Read the model definition and answer for the solid it produces. Units are mm, in the model's axes. A direction names the side the tool comes from. Round coordinates to 2 decimals unless told otherwise and drop trailing zeros. Loops run counter-clockwise (first coordinate to the right, second up) from the corner with the lowest first, then second, coordinate; pieces in that order, holes last. Notation, with made-up numbers: M 13.5,-17.5 L 31.5,-17.5 A18 cw 31.5,-7.5 Z; hole C 72,84 d8. An arc over 180 degrees is marked long. Answer as CSV lines item,"result".
```python
from build123d import *

# Parameters (mm, degrees)
SKETCH_1_R      = 8
EXTRUDE_1_DEPTH = 24
SKETCH_2_R      = 22
SKETCH_2_R_2    = 8
EXTRUDE_2_DEPTH = 18


with BuildPart() as part:
    # 草图1 → 凸台-拉伸1 (new body)
    with BuildSketch(Plane.XY):
        Circle(SKETCH_1_R)
        with BuildLine():
            Line((4.520101179, 2.361924075), (-4.833937562, 1.62574526))
            ThreePointArc((-4.833937562, 1.62574526), (0.400141388, -5.084278402), (4.520101179, 2.361924075))
        make_face(mode=Mode.SUBTRACT)
    extrude(amount=EXTRUDE_1_DEPTH)

    # 草图2 → 凸台-拉伸2 (add)
    with BuildSketch(Plane.XY):
        Circle(SKETCH_2_R)
        Circle(SKETCH_2_R_2, mode=Mode.SUBTRACT)
    extrude(amount=EXTRUDE_2_DEPTH)


solid = part.part
```
1) Find section C-C, the plane z = 5. Give the vertices of the cut face in (x, y).
Evaluation:
outline,"C 0,0 d44; hole M -4.83,1.63 A5.1 ccw long 4.52,2.36 Z"
2) Find section A-A, the plane y = 0. Give the vertices of the cut face in (x, z).
Evaluation:
outline,"M -22,0 L -5.1,0 L -5.1,24 L -8,24 L -8,18 L -22,18 Z; M 5.1,0 L 22,0 L 22,18 L 8,18 L 8,24 L 5.1,24 Z"
3) Find section D-D, the plane x = -6. Give the vertices of the cut face in (y, z), then the cut area to 3 significant figures.
Evaluation:
outline,"M -21.17,0 L 21.17,0 L 21.17,18 L 5.29,18 L 5.29,24 L -5.29,24 L -5.29,18 L -21.17,18 Z"
area,"825 mm^2"
4) Each of these flat-tipped pins is pushed along its axis until it touches: P1, Ø1, axis at y = 6, z = 17, coming from the +X side; P2, Ø1.5, axis at x = -10.5, z = 7, coming from the +Y side; P3, Ø5, axis at x = 15, y = 17, coming from the +Z side. Where does it stop, or does it pass through?
Evaluation:
P1,"stops at x = 21.3"
P2,"stops at y = 19.72"
P3,"stops at z = 18"
5) Straight lines are drawn through the part: line 1 (Z direction, x = -9.5, y = -4); line 2 (Y direction, x = 0, z = 5.5); line 3 (Y direction, x = -3, z = 20). For each, find the intervals that lie inside material, in ascending order.
Evaluation:
line 1,"z = 0 to 18"
line 2,"y = -22 to -5.1, 2.01 to 22"
line 3,"y = -7.42 to -4.12, 1.77 to 7.42"
6) Find section B-B, the plane x = 0. Give the vertices of the cut face in (y, z).
Evaluation:
outline,"M -22,0 L -5.1,0 L -5.1,24 L -8,24 L -8,18 L -22,18 Z; M 2.01,0 L 22,0 L 22,18 L 8,18 L 8,24 L 2.01,24 Z"
7) Determine the mould class of faces 3 (the cylindrical face through (-4.769, -21.477, 8.874)), 4 (the flat face through (0, 5, 0)), 5 (the flat face through (-0.1, 2, 11.8)) for opening direction X: released by +X, released by -X, zero draft, split by the parting line, or undercut.
Evaluation:
face 3,"split by the parting line"
face 4,"zero draft"
face 5,"undercut"
8) A tool of negligible diameter and unlimited length cuts with its end or side. For faces 1 (the cylindrical face through (-1.73, -7.81, 20.96)), 2 (the flat face through (-2, 2, 24)), from which of +Z, -Z, +X, -X, +Y, -Y can it reach the whole face along a straight path? Write none if from no direction.
Evaluation:
face 1,"+Z"
face 2,"+Z, +X, -X, +Y, -Y"
